```python
from build123d import *

# Parameters (mm, degrees)
ESQUISSE1_W                = 189
ESQUISSE1_H                = 130
BOSS_EXTRU_1_DEPTH         = 10
ESQUISSE2_W                = 30
ESQUISSE2_H                = 15
ENL_V_MAT_EXTRU_1_DEPTH    = 10
ESQUISSE3_W                = 10
ESQUISSE3_H                = 10
ENL_V_MAT_EXTRU_2_DEPTH    = 10
R_P_TITION_LIN_AIRE1_COUNT = 8
R_P_TITION_LIN_AIRE1_PITCH = 20
ESQUISSE4_R                = 5
BOSS_EXTRU_2_DEPTH         = 15
ESQUISSE5_R                = 5
BOSS_EXTRU_4_DEPTH         = 15


with BuildPart() as part:
    # Esquisse1 → Boss.-Extru.1 (new body)
    with BuildSketch(Plane(origin=(0, 0, 0), x_dir=(1, 0, 0), z_dir=(0, 1, 0))):
        with Locations((-94.5, 65)):
            Rectangle(ESQUISSE1_W, ESQUISSE1_H)
    extrude(amount=BOSS_EXTRU_1_DEPTH)

    # Esquisse2 → Enlèv. mat.-Extru.1 (cut)
    with BuildSketch(Plane(origin=(0, 10, 0), x_dir=(1, 0, 0), z_dir=(0, 1, 0))):
        with Locations((-174, 122.5)):
            Rectangle(ESQUISSE2_W, ESQUISSE2_H)
        with Locations((-174, 7.5)):
            Rectangle(ESQUISSE2_W, ESQUISSE2_H)
    extrude(amount=-ENL_V_MAT_EXTRU_1_DEPTH, mode=Mode.SUBTRACT)

    # Esquisse3 → Enlèv. mat.-Extru.2 (cut)
    with BuildSketch(Plane(origin=(0, 10, 0), x_dir=(1, 0, 0), z_dir=(0, 1, 0))):
        with Locations((-144, 125)):
            Rectangle(ESQUISSE3_W, ESQUISSE3_H)
        with Locations((-144, 5)):
            Rectangle(ESQUISSE3_W, ESQUISSE3_H)
    enl_v_mat_extru_2 = extrude(amount=-ENL_V_MAT_EXTRU_2_DEPTH, mode=Mode.SUBTRACT)

    # Répétition linéaire1: Enlèv. mat.-Extru.2 ×8
    with Locations(*[(i * R_P_TITION_LIN_AIRE1_PITCH, 0, 0) for i in range(1, R_P_TITION_LIN_AIRE1_COUNT)]):
        add(enl_v_mat_extru_2, mode=Mode.SUBTRACT)

    # Esquisse4 → Boss.-Extru.2 (add)
    with BuildSketch(Plane.XY.offset(-15)):
        with Locations((-184, 5)):
            Circle(ESQUISSE4_R)
    extrude(amount=BOSS_EXTRU_2_DEPTH)

    # Esquisse5 → Boss.-Extru.4 (add)
    with BuildSketch(Plane(origin=(0, 0, -115), x_dir=(-1, 0, 0), z_dir=(0, 0, -1))):
        with Locations((184, 5)):
            Circle(ESQUISSE5_R)
    extrude(amount=BOSS_EXTRU_4_DEPTH)


solid = part.part
```
Could you check a few things on this model? Use its own coordinates, in mm. A direction names the side the tool comes from. Round coordinates to 2 decimals unless told otherwise and drop trailing zeros. Order: outer loops, then holes, each group sorted by start corner. A loop starts at its lowest first (then second) coordinate and runs counter-clockwise, first axis right, second up. Notation, with made-up numbers: M 48,10.25 L 92,10.25 A29 ccw 92,38.25 Z; hole C 9,20.25 d1. An arc over 180 degrees is marked long. One line per question, with ' | ' between items. Start each with the question number.
(1) Thinking about a two-plate mould opening in X: for faces 5 (the face through (-59, 5, -125)), 6 (the face through (-188, 9, -15)), 7 (the face through (-189, 5, -64)), which applies, +X half, -X half, draft (parallel to the pull), parting line (faces both ways), or undercut?
(2) For faces 1 (the face through (-188, 2, -8)), 2 (the face through (-114, 5, -130)), 3 (the face through (-64, 5, -120)), 4 (the face through (-79, 5, -5)), which set-ups out of +Z, -Z, +X, -X, +Y, -Y let a thin tool reach every point of the face, with its end or its side?
(3) For P1, Ø1.5, axis at x = -82.5, y = 7.5, coming from the +Z side; P2, Ø3, axis at x = -21.5, y = 5.5, coming from the -Z side; P3, Ø3, axis at y = 7.5, z = -123.5, coming from the +X side; P4, Ø5.5, axis at x = -185.5, y = 8.5, coming from the +Z side, each with a flat end and sliding along its axis, tell me the tip position at first contact or that it passes through.
(4) Suppose I cut it at B-B on x = -166. List the corners of the cut face in (y, z) for me, then the cut area to 3 significant figures.
(5) Please list where these lines run through material, in increasing order: line 1 along Z through (x, y) = (-42, 5); line 2 along X through (y, z) = (4, -115.5); line 3 along X through (y, z) = (3.75, -14.5).
(6) Suppose I cut it at A-A on z = -7.5. Count the separate pieces of the cut face and the enclosed holes in it, then the cut area to 3 significant figures.
Geometry results:
1) face 5: undercut | face 6: draft | face 7: -X half
2) face 1: +Z | face 2: -Z, +X, -X, +Y, -Y | face 3: -Z, +Y, -Y | face 4: +Z, +Y, -Y
3) P1: z = -10 | P2: z = -120 | P3: x = -9 | P4: z = 0
4) outline: M 0,-115 L 10,-115 L 10,-15 L 0,-15 Z | area: 1,000 mm²
5) line 1: -120 to -10 | line 2: -188.9 to -179.1, -159 to 0 | line 3: -188.84 to -179.16, -159 to 0
6) separate pieces: 9 | enclosed holes: 0 | area: 879 mm²
